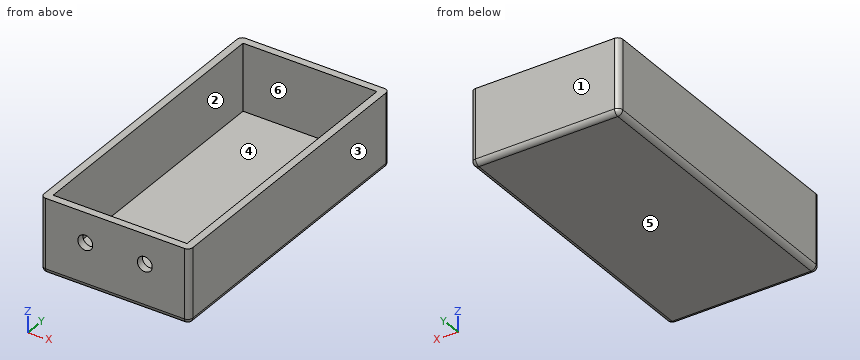
from build123d import *

# Parameters (mm, degrees)
F0_W     = 60
F0_H     = 120
F1_DEPTH = 30
F2_T     = -3
F3_R     = 2
F5_D     = 6
F5_DEPTH = 12
F6_R     = 2


with BuildPart() as f1:
    # F0 (on Top) → F1 (new body)
    with BuildSketch(Plane.XY):
        Rectangle(F0_W, F0_H)
    extrude(amount=F1_DEPTH)

    # F2
    f2_openings = [f1.faces().sort_by_distance(p)[0] for p in [
        (0, 0, 30),
    ]]
    offset(amount=F2_T, openings=f2_openings)

    # F3
    f3_edges = [f1.edges().sort_by_distance(p)[0] for p in [
        (30, -60, 15),
        (30, 60, 15),
        (-30, 60, 15),
        (-30, -60, 15),
    ]]
    fillet(f3_edges, radius=F3_R)

    # F5
    with Locations(Plane.XZ.offset(60)):
        with Locations((-12, 18.03771), (12, 18.03771)):
            Hole(F5_D / 2, depth=F5_DEPTH)

    # F6
    f6_edges = [f1.edges().sort_by_distance(p)[0] for p in [
        (30, 0, 0),
        (29.414214, -59.414214, 0),
        (29.414214, 59.414214, 0),
        (0, -60, 0),
        (0, 60, 0),
        (-29.414214, -59.414214, 0),
        (-29.414214, 59.414214, 0),
        (-30, 0, 0),
    ]]
    fillet(f6_edges, radius=F6_R)


solid = f1.part
Verification items for the finished model (mm, model axes). Face numbers are marked on the shaded views. A direction names the side the tool comes from. Give positions to 0.01 mm unless a question says otherwise; leave off trailing zeros. Write each loop counter-clockwise with the first axis right and the second up, starting at its lowest first coordinate (ties: lowest second). Pieces come first, ordered by that corner, then holes. Notation, with made-up numbers: M 4.5,-34.75 L 16.5,-34.75 A18 ccw 16.5,-23.75 Z; hole C -36.75,-32 d5. An arc over 180 degrees is marked long. Put each result on its own line as item: value. Start each with the question number.
1. Draft check along Y on the marked faces 1, 2, 3 and 4. Enter one of: +Y half, -Y half, draft (parallel to the pull), parting line (faces both ways), or undercut.
2. Section check B-B (x = 12). Record the cut outline in (y, z).
3. Scan lines: line 1 along Y through (x, z) = (5, 21.5); line 2 along X through (y, z) = (47, 10.75); line 3 along Z through (x, y) = (12, -58.25). Record each from-to range of solid material in increasing order. Write a range as [from, to].
4. Section check A-A (z = 8.25). Record the cut outline in (x, y), and give its area (3 significant figures).
5. Set-up check for the marked faces 5 and 6: record each of +Z, -Z, +X, -X, +Y, -Y from which the full face is reachable in a straight line by a thin tool's end or side.
6. Section check C-C (x = -20.5). Record the cut outline in (y, z).
7. Section check D-D (y = -47). Record the cut outline in (x, z).
Answer list:
1. face 1: +Y half
1. face 2: undercut
1. face 3: draft
1. face 4: undercut
2. outline: M -60,2 A2 ccw -58,0 L 58,0 A2 ccw 60,2 L 60,30 L 57,30 L 57,3 L -57,3 L -57,15.04 L -60,15.04 Z; M -60,21.04 L -57,21.04 L -57,30 L -60,30 Z
3. line 1: [-60, -57], [57, 60]
3. line 2: [-30, -27], [27, 30]
3. line 3: [0.02, 15.04], [21.04, 30]
4. outline: M -30,-58 A2 ccw -28,-60 L 28,-60 A2 ccw 30,-58 L 30,58 A2 ccw 28,60 L -28,60 A2 ccw -30,58 Z; hole M -27,-57 L 27,-57 L 27,57 L -27,57 Z
4. area: 1,040 mm2
5. face 5: -Z, +X, -X, +Y, -Y
5. face 6: +Z
6. outline: M -60,2 A2 ccw -58,0 L 58,0 A2 ccw 60,2 L 60,30 L 57,30 L 57,3 L -57,3 L -57,30 L -60,30 Z
7. outline: M -30,2 A2 ccw -28,0 L 28,0 A2 ccw 30,2 L 30,30 L 27,30 L 27,3 L -27,3 L -27,30 L -30,30 Z
